Input: part model. Units: mm. Frame: model coordinates. Coordinates: 2 decimals unless noted, no trailing zeros. Order: outer loops, then holes, each group sorted by start corner. A loop starts at its lowest first (then second) coordinate and runs counter-clockwise, first axis right, second up.
Autodesk Inventor part; units mm, degrees
ref_plane "YZ Plane" through (0, 0, 0) normal (1, 0, 0) x (0, 1, 0)
ref_plane "XZ Plane" through (0, 0, 0) normal (0, 1, 0) x (-1, 0, 0)
ref_plane "XY Plane" through (0, 0, 0) normal (0, 0, 1) x (1, 0, 0)
sketch "Sketch1" plane through (0, 0, 0) normal (0, 1, 0) x (-1, 0, 0)
  line L0 (50, 25) -> (-50, 25)
  line L1 (-50, 25) -> (-50, -25)
  line L2 (-50, -25) -> (50, -25)
  line L3 (50, -25) -> (50, 25)
  line L4 (50, 25) -> (-50, -25) construction
  line L5 (-50, 25) -> (50, -25) construction
  point P0 (0, 0)
  dimension "d0" = 100
  dimension "d1" = 50
extrude "Extrusion1" add sketch "Sketch1" along normal blind 3
fillet "Fillet1" radius 5 4 edges at (50, 1.5, 25) (50, 1.5, -25) (-50, 1.5, -25) (-50, 1.5, 25)
sketch "Sketch2" plane through (0, 3, 0) normal (0, 1, 0) x (1, 0, 0)
  arc A0 (-50, -20) -> (-45, -25) centre (-45, -20) ccw
  arc A1 (45, -25) -> (50, -20) centre (45, -20) ccw
  arc A2 (50, 20) -> (45, 25) centre (45, 20) ccw
  arc A3 (-45, 25) -> (-50, 20) centre (-45, 20) ccw
  point P0 (0, 0)
hole "Hole1" at (-45, 3, -20) at (-45, 3, 20) at (45, 3, 20) at (45, 3, -20) direction (0, -1, 0) diameter 4 end through all
properties part number "AcrylicLowerBottom" material "Acrylic, Clear"
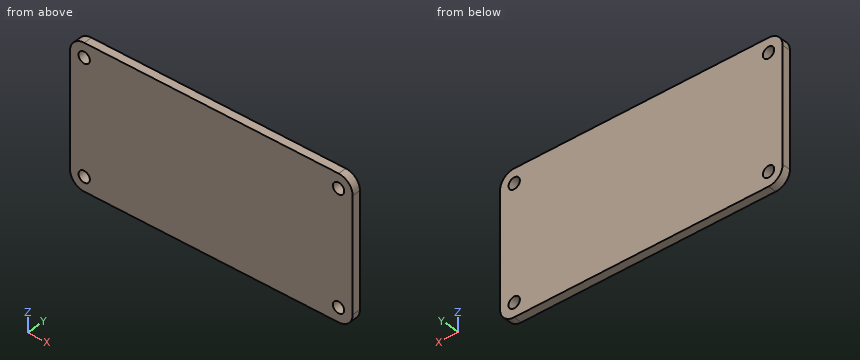
Item 1: Ray query, probe 1 along X at (y, z) = (0.95, -20); probe 2 along Z at (x, y) = (-45, 2.15). Return the intervals inside material, ascending.
Response values:
probe 1: x = -50 to -47, -43 to 43, 47 to 50
probe 2: z = -25 to -22, -18 to 18, 22 to 25
Item 2: Cut plane A-A on z = -21. Return loops of the section in (x, y).
Response values:
outline: (-49.9, 0) - (-46.73, 0) - (-46.73, 3) - (-49.9, 3) - close; (-43.27, 0) - (43.27, 0) - (43.27, 3) - (-43.27, 3) - close; (46.73, 0) - (49.9, 0) - (49.9, 3) - (46.73, 3) - close
Item 3: Pin query (flat end, axial travel): pin 1 Ø5 at (x, z) = (-45, 20) entering from -Y; pin 2 Ø3 at (x, z) = (-45, -20) entering from +Y. Return the tip coordinate at first contact, or that it passes through.
Response values:
pin 1: stops at y = 0
pin 2: passes through
